CAD build for the part. Positions are in the model's coordinates, mm. Face numbers are marked on the shaded views. A direction names the side the tool comes from. Give positions to 0.01 mm unless a question says otherwise; leave off trailing zeros. Order: outer loops, then holes, each group sorted by start corner. A loop starts at its lowest first (then second) coordinate and runs counter-clockwise, first axis right, second up.
Item 1: Band-saw the part on C-C on y = -7. Give the cut face in (x, z).
Item 2: Which spindle directions (+Z, -Z, +X, -X, +Y, -Y) get a long thin tool onto all of the face, cutting with end or side? Do the marked faces 4, 5, 6 and 7. Say none if no direction does.
Item 3: Wall check: L1, parallel to Z at x = -73.5, y = -42; L2, parallel to X at y = -39.5, z = -14.5; L3, parallel to Y at x = -50, z = 22.5. Give the ranges that are in metal, low to high.
Item 4: Two-plate mould, pull along X, no slides. Class the marked faces 1, 2 and 3: released by +X, released by -X, zero draft, split by the parting line, or undercut.
Item 5: Band-saw the part on B-B on z = 2.5. Give the cut face in (x, y), plus the area to 3 significant figures.
Item 6: Flat gauge pins, fed straight in: P1, Ø7.5, axis at y = -20.5, z = -3.5, coming from the +X side; P2, Ø4, axis at y = -9, z = -29.5, coming from the -X side; P3, Ø8.5, axis at x = -78.5, z = -37.5, coming from the -Y side; P4, Ø6.5, axis at x = -89.5, y = -17, coming from the -Z side. Where does each tip first touch, or does it go through?
Item 7: Band-saw the part on D-D on z = -18. Give the cut face in (x, y).
Item 8: Band-saw the part on A-A on x = 6. Give the cut face in (y, z), plus the area to 3 significant figures.
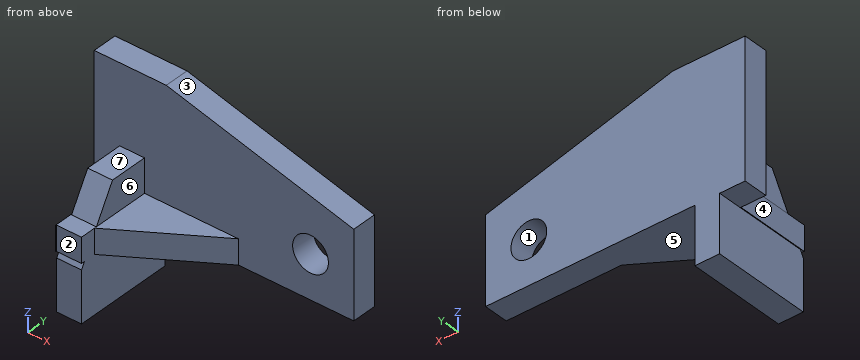
```python
from build123d import *

# Parameters (mm, degrees)
F0_R     = 7.874
F1_DEPTH = 10.922
F3_DEPTH = 10.922
F4_W     = 10.922
F4_H     = 50.8
F5_DEPTH = 44.45
F7_DEPTH = 25.4
F8_DEPTH = 0.254


with BuildPart() as f1:
    # F0 (on Front) → F1 (new body)
    with BuildSketch(Plane.XZ):
        Polygon((-95.0245559216, 40.9277565777), (-95.0245559216, -19.2702434223), (19.2754440784, -19.2702434223), (19.2754440784, 18.8085507425), (-63.2745559216, 40.9277565777), align=None)
        with Locations((0.2254440784, -0.2202434223)):
            Circle(F0_R, mode=Mode.SUBTRACT)
    extrude(amount=F1_DEPTH)

    # F2 (on face) → F3 (join)
    with BuildSketch(Plane(origin=(0, 0, -19.2702434223), x_dir=(1, 0, 0), z_dir=(0, 0, -1))):
        Polygon((-31.5245559216, 10.922), (-84.1025559216, 44.45), (-84.1025559216, 10.922), align=None)
    extrude(amount=-F3_DEPTH)

    # F4 (on Front) → F5 (join)
    with BuildSketch(Plane.XZ):
        with Locations((-78.3454434941, -18.9951797947)):
            Rectangle(F4_W, F4_H)
    extrude(amount=F5_DEPTH)

    # F6 (on face) → F7 (cut)
    with BuildSketch(Plane(origin=(-83.8064434941, 0, 0), x_dir=(0, -1, 0), z_dir=(-1, 0, 0))):
        Polygon((44.45, 6.4048202053), (27.814247327, 6.4048202053), (36.3319325837, -8.3482434223), (44.261174684, -8.3482434223), (44.261174684, -19.2702434223), (42.6377522238, -19.2702434223), (44.3853547532, -22.2971797947), align=None)
    extrude(amount=-F7_DEPTH, mode=Mode.SUBTRACT)

    # F8 (cut): a face of the model
    f8_faces = [f1.faces().sort_by_distance(p)[0] for p in [
        (-78.3454434941, -44.45, -18.9951797947),
    ]]
    extrude(f8_faces, amount=-F8_DEPTH, mode=Mode.SUBTRACT)


solid = f1.part
```
The answers:
1. outline: (-95.02, -19.27) - (-83.81, -19.27) - (-83.81, -44.4) - (-72.88, -44.4) - (-72.88, -19.27) - (19.28, -19.27) - (19.28, 18.81) - (-63.27, 40.93) - (-95.02, 40.93) - close; hole circle Ø15.75 at (0.23, -0.22)
2. face 4: +Z, -Z, -X, -Y
2. face 5: -Z, +X, +Y, -Y
2. face 6: +Z, +X, -Y
2. face 7: +Z, +X, -X, -Y
3. L1: z = -44.4 to -8.35
3. L2: x = -84.1 to -72.88
3. L3: y = -10.92 to 0
4. face 1: undercut
4. face 2: zero draft
4. face 3: released by +X
5. outline: (-95.02, -10.92) - (-83.81, -10.92) - (-83.81, -30.07) - (-72.88, -30.07) - (-72.88, -10.92) - (-7.16, -10.92) - (-7.16, 0) - (-95.02, 0) - close; (7.61, -10.92) - (19.28, -10.92) - (19.28, 0) - (7.61, 0) - close
5. area: 1,300 mm2
6. P1: stops at x = -72.88
6. P2: stops at x = -83.81
6. P3: stops at y = -44.2
6. P4: passes through
7. outline: (-95.02, -10.92) - (-84.1, -10.92) - (-84.1, -44.45) - (-83.81, -44.26) - (-83.81, -44.2) - (-72.88, -44.2) - (-72.88, -37.3) - (-31.52, -10.92) - (19.28, -10.92) - (19.28, 0) - (-95.02, 0) - close
8. outline: (-10.92, -19.27) - (0, -19.27) - (0, -5.57) - (-10.92, -5.57) - close; (-10.92, 5.13) - (0, 5.13) - (0, 22.37) - (-10.92, 22.37) - close
8. area: 338 mm2
